The listing builds one solid part. Answer for the finished solid, in the listing's coordinates (mm). Give positions to 0.01 mm unless a question says otherwise; leave off trailing zeros. Loops run counter-clockwise (first coordinate to the right, second up) from the corner with the lowest first, then second, coordinate; pieces in that order, holes last. Notation, with made-up numbers: (50.5, 40) - (54.5, 40) arc R14 cw to (54.5, 56) - close; hole circle Ø5 at (0, -36.5). An arc over 180 degrees is marked (long way). Write item = value, one per line. Start each with the question number.
1) Consider probe 1 along Y at (x, z) = (10.25, -13.2); probe 2 along Z at (x, y) = (11.5, 152.4); probe 3 along Y at (x, z) = (10.25, -38.6). Determine where each line is inside the solid, lowest interval first.
2) The part is cut by section C-C on y = 152.4. Write down the section's boundary in (x, z) (3 decimals).
3) The mould has two halves that part along Z. Classify faces 1 (the cylindrical face through (9.649, 148.333, -38.066)), 2 (the flat face through (0, 45, -140)), 3 (the cylindrical face through (9.66, 3.09, -140.93)): +Z half, -Z half, draft (parallel to the pull), parting line (faces both ways), or undercut.
4) The part is cut by section D-D on z = -13.2. Write down the section's boundary in (x, y) (3 decimals), plus the area to 3 significant figures.
5) Flat-ended cylindrical pins translate along their axes: P1, Ø1.5, axis at x = 14, y = -9.5, coming from the +Z side; P2, Ø4, axis at x = 9, z = -102, coming from the -Y side; P3, Ø5, axis at x = 7, z = -93.5, coming from the -Y side. Find the tip coordinate at first contact, or state that the pin passes through.
6) The part is cut by section A-A on x = 3.5. Write down the section's boundary in (y, z) (1 decimal), plus the area to 3 significant figures.
7) The part is cut by section B-B on z = -99.5. Write down the section's boundary in (x, y), plus the area to 3 significant figures.
from build123d import *

# Parameters (mm, degrees)
SKETCH1_W                         = 19.05
SKETCH1_H                         = 50.8
REVOLVE_THIN1_ANGLE               = 180
SKETCH81_W                        = 0.5
SKETCH81_H                        = 430
EXTRUDE1_DEPTH                    = 20.05
F_5_16_CLEARANCE_HOLE1_AT_2_COUNT = 2
F_5_16_CLEARANCE_HOLE1_AT_2_PITCH = 25.4
F_5_16_CLEARANCE_HOLE1_AT_3_COUNT = 2
F_5_16_CLEARANCE_HOLE1_AT_3_PITCH = 304.8
F_5_16_CLEARANCE_HOLE1_AT_4_COUNT = 2
F_5_16_CLEARANCE_HOLE1_AT_4_PITCH = 305.856502301


with BuildPart() as part:
    # Sketch1 → Revolve-Thin1 (revolve)
    with BuildSketch(Plane.XY):
        with Locations((9.525, 166.3625)):
            Rectangle(SKETCH1_W, SKETCH1_H)
    revolve(axis=Axis((0, 0, 0), (-1, 0, 0)), revolution_arc=REVOLVE_THIN1_ANGLE)

    # Sketch81 → Extrude1 (cut, through all)
    with BuildSketch(Plane(origin=(0, 0, 0), x_dir=(0, 0, -1), z_dir=(1, 0, 0))):
        with Locations((0.25, 0)):
            Rectangle(SKETCH81_W, SKETCH81_H)
    extrude(amount=EXTRUDE1_DEPTH, mode=Mode.SUBTRACT)

    # Sketch82 → 5_16 Clearance Hole1 (revolve, cut)
    with BuildSketch(Plane(origin=(19.05, 152.4, -38.6), x_dir=(0, 0, -1), z_dir=(0, 1, 0))):
        Polygon((0, 0), (0, 19.05), (4.7371, 19.05), (4.1021, 18.415), (4.1021, 0.635), (4.7371, 0), align=None)
    f_5_16_clearance_hole1 = revolve(axis=Axis((25.4, 152.4, -38.6), (-1, 0, 0)), mode=Mode.SUBTRACT)

    # 5_16 Clearance Hole1 at 2: 5_16 Clearance Hole1 ×2
    with Locations(*[(0, 0, i * F_5_16_CLEARANCE_HOLE1_AT_2_PITCH) for i in range(1, F_5_16_CLEARANCE_HOLE1_AT_2_COUNT)]):
        add(f_5_16_clearance_hole1, mode=Mode.SUBTRACT)

    # 5_16 Clearance Hole1 at 3: 5_16 Clearance Hole1 ×2
    with Locations(*[(0, -i * F_5_16_CLEARANCE_HOLE1_AT_3_PITCH, 0) for i in range(1, F_5_16_CLEARANCE_HOLE1_AT_3_COUNT)]):
        add(f_5_16_clearance_hole1, mode=Mode.SUBTRACT)

    # 5_16 Clearance Hole1 at 4: 5_16 Clearance Hole1 ×2
    with Locations(*[Vector(0, -0.996545758, 0.08304548) * (i * F_5_16_CLEARANCE_HOLE1_AT_4_PITCH) for i in range(1, F_5_16_CLEARANCE_HOLE1_AT_4_COUNT)]):
        add(f_5_16_clearance_hole1, mode=Mode.SUBTRACT)


solid = part.part
Answer below:
q1.probe_1 = -191.31 to -156.5, -148.3 to -140.34, 140.34 to 148.3, 156.5 to 191.31
q1.probe_2 = -116.39 to -42.7, -34.5 to -17.3, -9.1 to -0.5
q1.probe_3 = -187.84 to -156.5, -148.3 to -135.57, 135.57 to 148.3, 156.5 to 187.84
q2.outline = (0, -116.392) - (19.05, -116.392) - (19.05, -43.337) - (18.415, -42.702) - (0.635, -42.702) - (0, -43.337) - close; (0, -33.863) - (0.635, -34.498) - (18.415, -34.498) - (19.05, -33.863) - (19.05, -17.937) - (18.415, -17.302) - (0.635, -17.302) - (0, -17.937) - close; (0, -8.463) - (0.635, -9.098) - (18.415, -9.098) - (19.05, -8.463) - (19.05, -0.5) - (0, -0.5) - close
q3.face_1 = undercut
q3.face_2 = draft
q3.face_3 = +Z half
q4.outline = (0, -191.308) - (19.05, -191.308) - (19.05, -157.137) - (18.415, -156.502) - (0.635, -156.502) - (0, -157.137) - close; (0, -147.663) - (0.635, -148.298) - (18.415, -148.298) - (19.05, -147.663) - (19.05, -140.343) - (0, -140.343) - close; (0, 140.343) - (19.05, 140.343) - (19.05, 147.663) - (18.415, 148.298) - (0.635, 148.298) - (0, 147.663) - close; (0, 157.137) - (0.635, 156.502) - (18.415, 156.502) - (19.05, 157.137) - (19.05, 191.308) - (0, 191.308) - close
q4.area = 1,630 mm2
q5.P1 = -140.59
q5.P2 = -163.62
q5.P3 = -168.8
q6.outline = (-191.8, -0.5) arc R191.8 ccw to (191.8, -0.5) - (141, -0.5) arc R141 cw to (-141, -0.5) - close; hole circle Ø8.2 at (-152.4, -38.6); hole circle Ø8.2 at (-152.4, -13.2); hole circle Ø8.2 at (152.4, -38.6); hole circle Ø8.2 at (152.4, -13.2)
q6.area = 26,300 mm2
q7.outline = (0, -163.93) - (19.05, -163.93) - (19.05, -99.85) - (0, -99.85) - close; (0, 99.85) - (19.05, 99.85) - (19.05, 163.93) - (0, 163.93) - close
q7.area = 2,440 mm2
